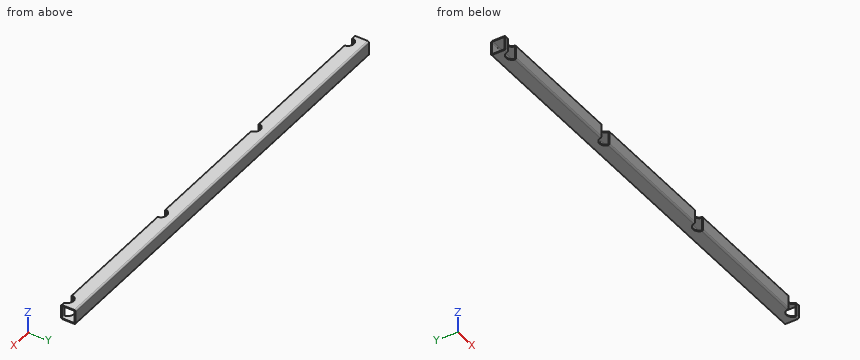
from build123d import *

# Parameters (mm, degrees)
EXTRUDE_1_DEPTH      = 884.980118
EXTRUDE_1_DEPTH_BACK = 20
OTHER_START          = -15
OTHER_2_DEPTH        = 30


# Read off the part's stored shape, not the designer's step: Полость2
with BuildPart() as part:
    # Эскиз1 → Бобышка-Вытянуть1 (new, two sides: drawn at the far end of the back side and taken through both)
    with BuildSketch(Plane(origin=(0, 0, 0), x_dir=(0, 0, -1), z_dir=(1, 0, 0)).offset(-EXTRUDE_1_DEPTH_BACK)):
        with BuildLine():
            Line((-12, 30), (12, 30))
            ThreePointArc((12, 30), (14.121320344, 29.121320344), (15, 27))
            Line((15, 27), (15, 3))
            ThreePointArc((15, 3), (14.121320344, 0.878679656), (12, 0))
            Line((12, 0), (-12, 0))
            ThreePointArc((-12, 0), (-14.121320344, 0.878679656), (-15, 3))
            Line((-15, 3), (-15, 27))
            ThreePointArc((-15, 27), (-14.121320344, 29.121320344), (-12, 30))
        make_face()
        with BuildLine():
            Line((-11, 28), (11, 28))
            ThreePointArc((11, 28), (12.414213562, 27.414213562), (13, 26))
            Line((13, 26), (13, 4))
            ThreePointArc((13, 4), (12.414213562, 2.585786438), (11, 2))
            Line((11, 2), (-11, 2))
            ThreePointArc((-11, 2), (-12.414213562, 2.585786438), (-13, 4))
            Line((-13, 4), (-13, 26))
            ThreePointArc((-13, 26), (-12.414213562, 27.414213562), (-11, 28))
        make_face(mode=Mode.SUBTRACT)
    extrude(amount=EXTRUDE_1_DEPTH + EXTRUDE_1_DEPTH_BACK)

    # Полость2 outline → Полость2 (cut)
    with BuildSketch(Plane.XY.offset(OTHER_START)):
        with BuildLine():
            Line((852.480118087, -4.981e-06), (877.480118087, -4.981e-06))
            ThreePointArc((877.480118087, -4.981e-06), (877.439793915, 1.003233908), (877.319080766, 2))
            Line((877.319080766, 2), (852.641155408, 2))
            ThreePointArc((852.641155408, 2), (852.52044226, 1.003233908), (852.480118087, -4.981e-06))
        make_face()
        with BuildLine():
            Line((852.641155408, 2), (877.319080766, 2))
            ThreePointArc((877.319080766, 2), (864.980118087, 12.5), (852.641155408, 2))
        make_face()
        with BuildLine():
            Line((564.153412058, -4.981e-06), (589.153412058, -4.981e-06))
            ThreePointArc((589.153412058, -4.981e-06), (589.113087885, 1.003233908), (588.992374737, 2))
            Line((588.992374737, 2), (564.314449379, 2))
            ThreePointArc((564.314449379, 2), (564.193736231, 1.003233908), (564.153412058, -4.981e-06))
        make_face()
        with BuildLine():
            Line((564.314449379, 2), (588.992374737, 2))
            ThreePointArc((588.992374737, 2), (576.653412058, 12.5), (564.314449379, 2))
        make_face()
        with BuildLine():
            Line((275.826706029, -4.981e-06), (300.826706029, -4.981e-06))
            ThreePointArc((300.826706029, -4.981e-06), (300.786381856, 1.003233908), (300.665668708, 2))
            Line((300.665668708, 2), (275.98774335, 2))
            ThreePointArc((275.98774335, 2), (275.867030202, 1.003233908), (275.826706029, -4.981e-06))
        make_face()
        with BuildLine():
            Line((275.98774335, 2), (300.665668708, 2))
            ThreePointArc((300.665668708, 2), (288.326706029, 12.5), (275.98774335, 2))
        make_face()
        with BuildLine():
            Line((-12.5, -4.981e-06), (12.5, -4.981e-06))
            ThreePointArc((12.5, -4.981e-06), (12.459675827, 1.003233908), (12.338962679, 2))
            Line((12.338962679, 2), (-12.338962679, 2))
            ThreePointArc((-12.338962679, 2), (-12.459675827, 1.003233908), (-12.5, -4.981e-06))
        make_face()
        with BuildLine():
            Line((-12.338962679, 2), (12.338962679, 2))
            ThreePointArc((12.338962679, 2), (0, 12.5), (-12.338962679, 2))
        make_face()
    extrude(amount=OTHER_2_DEPTH, mode=Mode.SUBTRACT)


solid = part.part
Work out the finished part from the listing and answer in its coordinate system (mm). Give positions to 0.01 mm unless a question says otherwise; leave off trailing zeros. Loops run counter-clockwise (first coordinate to the right, second up) from the corner with the lowest first, then second, coordinate; pieces in that order, holes last. Notation, with made-up numbers: (-31.75, 65) -> (-4.75, 65) arc R16 ccw to (-4.75, 72) -> close; hole circle Ø2 at (12.25, -37). An arc over 180 degrees is marked (long way). Use a Markdown table: item, result. Add a question column.
1. Section B-B on x = 518.5 is taken. Determine the outline of the cut face in (y, z).
2. Section A-A on z = 3 is taken. Determine the outline of the cut face in (x, y).
3. Find the intervals of material crossed by probe 1 along X at (y, z) = (1, 0.5); probe 2 along Z at (x, y) = (297, 19.5); probe 3 along Y at (x, z) = (274, -2), in increasing order.
4. Section C-C on y = 18 is taken. Determine the outline of the cut face in (x, z).
5. A flat-ended cylindrical pin translates along its axis: pin 1 Ø5 at (y, z) = (24.5, 5.5) entering from -X. Find the tip coordinate at first contact, or state that the pin passes through.
Results below:
| question | item | result |
|---|---|---|
| 1 | outline | (0, -12) arc R3 ccw to (3, -15) -> (27, -15) arc R3 ccw to (30, -12) -> (30, 12) arc R3 ccw to (27, 15) -> (3, 15) arc R3 ccw to (0, 12) -> close; hole (2, -11) arc R2 ccw to (4, -13) -> (26, -13) arc R2 ccw to (28, -11) -> (28, 11) arc R2 ccw to (26, 13) -> (4, 13) arc R2 ccw to (2, 11) -> close |
| 2 | outline | (-20, 0) -> (-12.5, 0) arc R12.5 cw to (-12.34, 2) -> (-20, 2) -> close; (-20, 28) -> (884.98, 28) -> (884.98, 30) -> (-20, 30) -> close; (12.34, 2) arc R12.5 cw to (12.5, 0) -> (275.83, 0) arc R12.5 cw to (275.99, 2) -> close; (300.67, 2) arc R12.5 cw to (300.83, 0) -> (564.15, 0) arc R12.5 cw to (564.31, 2) -> close; (588.99, 2) arc R12.5 cw to (589.15, 0) -> (852.48, 0) arc R12.5 cw to (852.64, 2) -> close; (877.32, 2) arc R12.5 cw to (877.48, 0) -> (884.98, 0) -> (884.98, 2) -> close |
| 3 | probe 1 | x = -20 to -12.46, 12.46 to 275.87, 300.79 to 564.19, 589.11 to 852.52, 877.44 to 884.98 |
| 3 | probe 2 | z = -15 to -13, 13 to 15 |
| 3 | probe 3 | y = 0 to 2, 28 to 30 |
| 4 | outline | (-20, -15) -> (884.98, -15) -> (884.98, -13) -> (-20, -13) -> close; (-20, 13) -> (884.98, 13) -> (884.98, 15) -> (-20, 15) -> close |
| 5 | pin 1 | passes through |
